from build123d import *

# Parameters (mm, degrees)
SKETCH1_R           = 1.5
SKETCH1_R_2         = 2
BOSS_EXTRUDE1_DEPTH = 3


with BuildPart() as part:
    # Sketch1 → Boss-Extrude1 (new body)
    with BuildSketch(Plane(origin=(0, 0, 0), x_dir=(1, 0, 0), z_dir=(0, 1, 0))):
        with BuildLine():
            Line((6.5, 0), (73.5, 0))
            ThreePointArc((73.5, 0), (78.096194078, 1.903805922), (80, 6.5))
            Line((80, 6.5), (80, 23))
            Line((80, 23), (69, 23))
            Line((69, 23), (69, 57))
            Line((69, 57), (80, 57))
            Line((80, 57), (80, 73.5))
            ThreePointArc((80, 73.5), (78.096194078, 78.096194078), (73.5, 80))
            Line((73.5, 80), (6.5, 80))
            ThreePointArc((6.5, 80), (1.903805922, 78.096194078), (0, 73.5))
            Line((0, 73.5), (0, 57))
            Line((0, 57), (11, 57))
            Line((11, 57), (11, 23))
            Line((11, 23), (0, 23))
            Line((0, 23), (0, 6.5))
            ThreePointArc((0, 6.5), (1.903805922, 1.903805922), (6.5, 0))
        make_face()
        with Locations(Location((16, 54, 0), (0, 0, 270))):
            Circle(SKETCH1_R, mode=Mode.SUBTRACT)
        with Locations(Location((16, 28, 0), (0, 0, 270))):
            Circle(SKETCH1_R, mode=Mode.SUBTRACT)
        with Locations(Location((64, 28, 0), (0, 0, 90))):
            Circle(SKETCH1_R, mode=Mode.SUBTRACT)
        with Locations(Location((64, 54, 0), (0, 0, 90))):
            Circle(SKETCH1_R, mode=Mode.SUBTRACT)
        with Locations(Location((23, 53.5, 0), (0, 0, 270))):
            Circle(SKETCH1_R_2, mode=Mode.SUBTRACT)
        with Locations(Location((23, 26.5, 0), (0, 0, 270))):
            Circle(SKETCH1_R_2, mode=Mode.SUBTRACT)
        with Locations(Location((57, 26.5, 0), (0, 0, 90))):
            Circle(SKETCH1_R_2, mode=Mode.SUBTRACT)
        with Locations(Location((57, 53.5, 0), (0, 0, 90))):
            Circle(SKETCH1_R_2, mode=Mode.SUBTRACT)
        with Locations(Location((40, 69, 0), (0, 0, 270))):
            Circle(SKETCH1_R, mode=Mode.SUBTRACT)
        with Locations(Location((40, 11, 0), (0, 0, 90))):
            Circle(SKETCH1_R, mode=Mode.SUBTRACT)
    extrude(amount=BOSS_EXTRUDE1_DEPTH)


solid = part.part
Could you check a few things on this model? Use its own coordinates, in mm. A direction names the side the tool comes from. Give positions to 0.01 mm unless a question says otherwise; leave off trailing zeros. Order: outer loops, then holes, each group sorted by start corner. A loop starts at its lowest first (then second) coordinate and runs counter-clockwise, first axis right, second up. Notation, with made-up numbers: (14.25, -5) - (55.25, -5) arc R15 ccw to (55.25, 13) - close; hole circle Ø9 at (-31.75, 45.25). An arc over 180 degrees is marked (long way). One line per item, written item: value. Start each with the question number.
1. Thinking about a two-plate mould opening in X: for faces 4 (the face through (78.045, 1.479, -1.854)), 5 (the face through (5, 1, -57)), 6 (the face through (62.735, 1.479, -54.806)), which applies, +X half, -X half, draft (parallel to the pull), parting line (faces both ways), or undercut?
2. For P1, Ø1.5, axis at y = 1, z = -48.5, coming from the -X side, with a flat end and sliding along its axis, tell me the tip position at first contact or that it passes through.
3. Imagine slicing it at B-B on z = -69. List the corners of the cut face in (x, y) for me.
4. Imagine slicing it at D-D on x = 64. List the corners of the cut face in (y, z) for me.
5. Imagine slicing it at A-A on x = 23. List the corners of the cut face in (y, z) for me.
6. For faces 1 (the face through (78.146, 1.479, -78.045)), 2 (the face through (74, 1, -57)), 3 (the face through (6, 1, -23)), which set-ups out of +Z, -Z, +X, -X, +Y, -Y let a thin tool reach every point of the face, with its end or its side?
7. Imagine slicing it at C-C on y = 0.9. Give the number of separate pieces and of enclosed holes in the cut face, plus the area to 3 significant figures.
8. If I drill on probe 1 along Z at (x, y) = (57, 1.2); probe 2 along X at (y, z) = (0.85, -69); probe 3 along X at (y, z) = (2.3, -53.5), over which ranges is the centre line in solid material (lowest first)?
Values:
1. face 4: +X half
1. face 5: draft
1. face 6: undercut
2. P1: x = 11
3. outline: (0, 0) - (38.5, 0) - (38.5, 3) - (0, 3) - close; (41.5, 0) - (80, 0) - (80, 3) - (41.5, 3) - close
4. outline: (0, -80) - (3, -80) - (3, -55.5) - (0, -55.5) - close; (0, -52.5) - (3, -52.5) - (3, -29.5) - (0, -29.5) - close; (0, -26.5) - (3, -26.5) - (3, 0) - (0, 0) - close
5. outline: (0, -80) - (3, -80) - (3, -55.5) - (0, -55.5) - close; (0, -51.5) - (3, -51.5) - (3, -28.5) - (0, -28.5) - close; (0, -24.5) - (3, -24.5) - (3, 0) - (0, 0) - close
6. face 1: -Z, +X, +Y, -Y
6. face 2: +X, +Y, -Y
6. face 3: -X, +Y, -Y
7. separate pieces: 1
7. enclosed holes: 10
7. area: 5,520 mm²
8. probe 1: -80 to -55.5, -51.5 to -28.5, -24.5 to 0
8. probe 2: 0 to 38.5, 41.5 to 80
8. probe 3: 11 to 14.59, 17.41 to 21, 25 to 55, 59 to 62.59, 65.41 to 69
